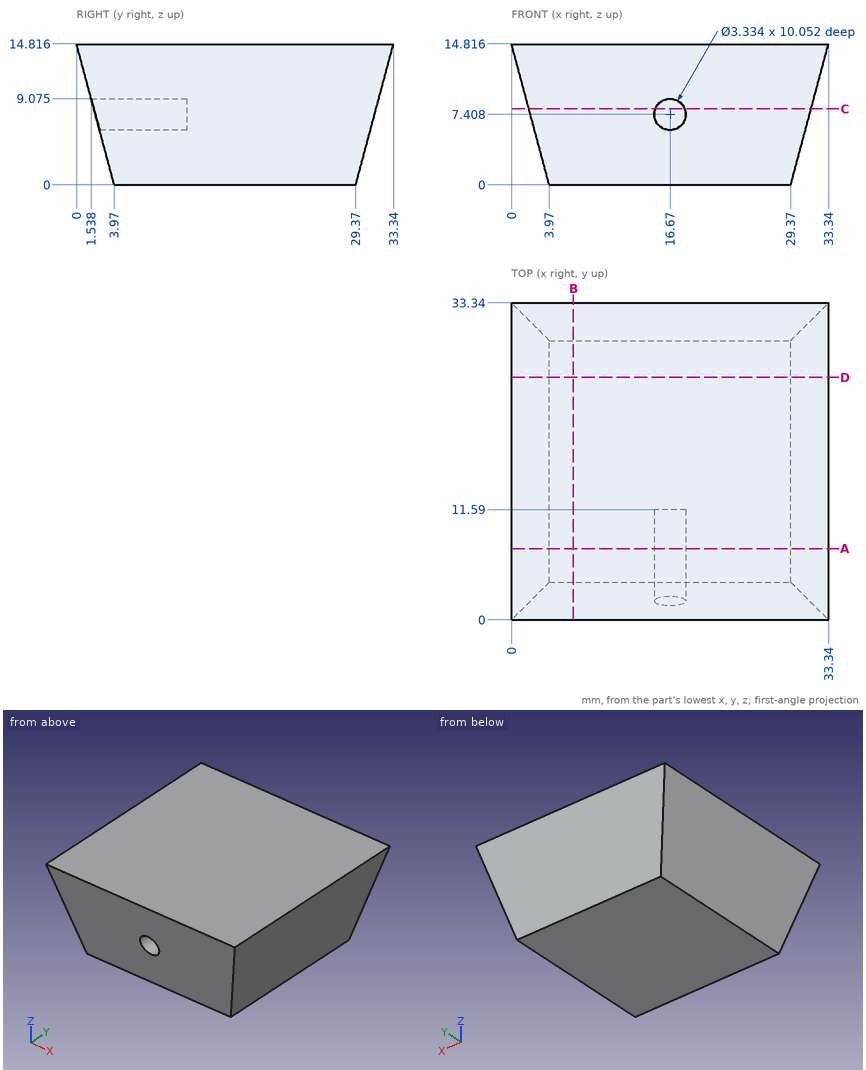
Check sheet for the drawn part. Datum: minimum x, y, z corner. Units: mm. Give positions to 0.01 mm unless a question says otherwise; leave off trailing zeros. Order: outer loops, then holes, each group sorted by start corner. A loop starts at its lowest first (then second) coordinate and runs counter-clockwise, first axis right, second up. Notation, with made-up numbers: (10.25, 50.5) - (39.25, 50.5) arc R29 ccw to (39.25, 88.5) - close; hole circle Ø7 at (49.25, -6.75). An arc over 180 degrees is marked (long way). Write item = value, one per line. Start each with the question number.
1) Section check C-C (z = 8). Enter the section's corners in (x, y).
2) Gauge pin test, flat ends, axial feed: pin 1 Ø2 at (x, z) = (16.67, 7.41) entering from -Y; pin 2 Ø8 at (x, z) = (12.5, 8) entering from +Y (1 decimal); pin 3 Ø6 at (x, y) = (18.5, 17.5) entering from -Z; pin 4 Ø5 at (y, z) = (12, 7) entering from -X (1 decimal). Record the tip position at first contact, or that the pin passes through.
3) Scan lines: L1, parallel to Y at x = 28, z = 10; L2, parallel to Y at x = 16.5, z = 3.5; L3, parallel to X at y = 22.5, z = 13.25. Record each from-to range of solid material in increasing order.
4) Section check A-A (y = 7.5). Enter the section's corners in (x, z) (1 decimal).
5) Section check B-B (x = 6.5). Enter the section's corners in (y, z) (1 decimal), then the cut area to 3 significant figures.
Geometry check:
q1.outline = (1.83, 1.83) - (15.11, 1.83) - (15.11, 11.59) - (18.23, 11.59) - (18.23, 1.83) - (31.51, 1.83) - (31.51, 31.51) - (1.83, 31.51) - close
q2.pin_1 = 11.59
q2.pin_2 = 32.6
q2.pin_3 = 0
q2.pin_4 = 1.4
q3.L1 = 1.29 to 32.05
q3.L2 = 3.03 to 30.31
q3.L3 = 0.42 to 32.92
q4.outline = (0, 14.8) - (4, 0) - (29.4, 0) - (33.3, 14.8) - close; hole circle Ø3.3 at (16.7, 7.4)
q5.outline = (0, 14.8) - (4, 0) - (29.4, 0) - (33.3, 14.8) - close
q5.area = 435 mm2
